from build123d import *

# Parameters (mm, degrees)
BOX_W        = 20
BOX_H        = 5
BOX_DEPTH    = 200
SKETCH_R     = 2.5
POCKET_DEPTH = 5


with BuildPart() as part:
    # Box → Box (new body)
    with BuildSketch(Plane.XY):
        with Locations((10, 2.5)):
            Rectangle(BOX_W, BOX_H)
    extrude(amount=BOX_DEPTH)

    # Sketch (on Face3 of Box) → Pocket (cut)
    with BuildSketch(Plane.XZ):
        with Locations((10, 15)):
            Circle(SKETCH_R)
    extrude(amount=-POCKET_DEPTH, mode=Mode.SUBTRACT)


solid = part.part
Model file for the job. Use its own axes, mm. Give positions to 0.01 mm unless a question says otherwise; leave off trailing zeros. Order: outer loops, then holes, each group sorted by start corner. A loop starts at its lowest first (then second) coordinate and runs counter-clockwise, first axis right, second up. Notation, with made-up numbers: (-21.5, 42.5) - (-14.5, 42.5) arc R21 ccw to (-14.5, 48.5) - close; hole circle Ø7 at (-1.75, 50). An arc over 180 degrees is marked (long way). Write item = value, one per line. Start each with the question number.
1. Two-plate mould, pull along X, no slides. Class faces 1 (the cylindrical face through (9.46, 2.46, 12.56)), 2 (the flat face through (0, 2, 99)), 3 (the flat face through (10, 5, 99)): pulls with the +X half, pulls with the -X half, needs draft (parallel to the pull), parting line crosses it, or undercut.
2. Cut at B-B, the plane x = 10. List the corners of the cut face in (y, z), and give its area (3 significant figures).
3. Probe line 1 along Z through (x, y) = (10, 1.5); line 2 along Z through (x, y) = (10.5, 3.2). List the from-to ranges inside material, lowest first.
4. Cut at A-A, the plane z = 15. List the corners of the cut face in (x, y).
Taken from the geometry:
q1.face_1 = undercut
q1.face_2 = pulls with the -X half
q1.face_3 = needs draft
q2.outline = (0, 0) - (5, 0) - (5, 12.5) - (0, 12.5) - close; (0, 17.5) - (5, 17.5) - (5, 200) - (0, 200) - close
q2.area = 975 mm²
q3.line_1 = 0 to 12.5, 17.5 to 200
q3.line_2 = 0 to 12.55, 17.45 to 200
q4.outline = (0, 0) - (7.5, 0) - (7.5, 5) - (0, 5) - close; (12.5, 0) - (20, 0) - (20, 5) - (12.5, 5) - close
